Input: dimensioned drawing with shaded views. Units: mm. Origin: part minimum x, y, z. A direction names the side the tool comes from. Round coordinates to 2 decimals unless told otherwise and drop trailing zeros. Order: outer loops, then holes, each group sorted by start corner. A loop starts at its lowest first (then second) coordinate and runs counter-clockwise, first axis right, second up.
Item 1: Mould query, pull axis Z, two halves, no side actions, for the marked faces 3, 4 and 5. Classes: released by +Z, released by -Z, zero draft, split by the parting line, or undercut.
Item 2: Cut plane B-B on y = 38.1. Output: boundary loops of the cut face in (x, z), then the cut area to 3 significant figures.
Item 3: Cut plane D-D on z = 38.1. Output: boundary loops of the cut face in (x, y).
Item 4: Cut plane C-C on x = 22.86. Output: boundary loops of the cut face in (y, z), then the cut area to 3 significant figures.
Item 5: Cut plane A-A on z = 10.16. Output: boundary loops of the cut face in (x, y), then the cut area to 3 significant figures.
Item 6: Line query: L1, parallel to X at y = 6, z = 10; L2, parallel to Z at x = 78.74, y = 2.75; L3, parallel to X at y = 6.5, z = 67. Output: solid intervals per line, ascending.
Item 7: First-contact query: pin 1 (3 mm diameter, centred on x = 10.5, y = 66.5, fed in from +Z); pin 2 (2.5 mm diameter, centred on x = 22.86, z = 10.16, fed in from +Y); pin 3 (5 mm diameter, centred on x = 79, z = 63.5, fed in from +Y). Flat tips, straight axial feed; report the tip coordinate or a pass-through.
Item 8: Reachability of the marked faces 1 and 2 from +Z, -Z, +X, -X, +Y, -Y: full face, straight path, thin tool, end or side. Return the list, or none.
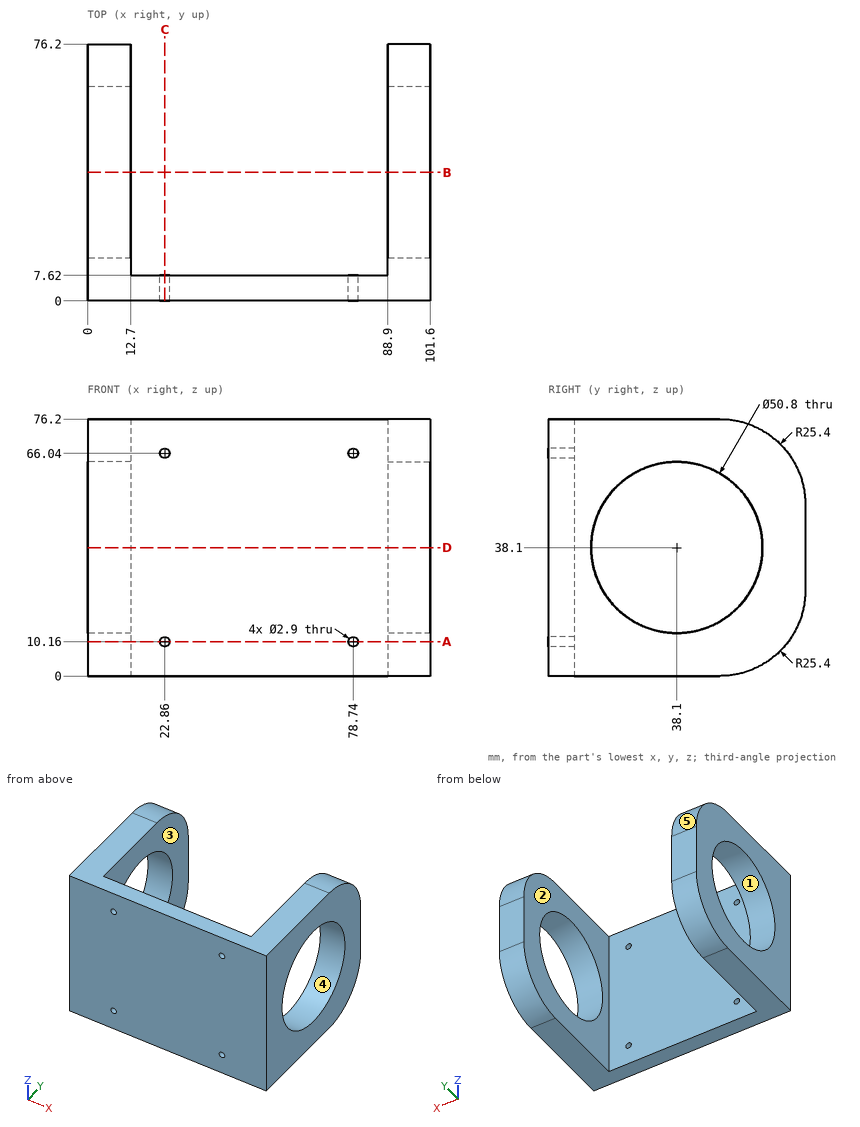
From the geometry:
1. face 3: zero draft
1. face 4: undercut
1. face 5: released by +Z
2. outline: (0, 0) - (12.7, 0) - (12.7, 12.7) - (0, 12.7) - close; (0, 63.5) - (12.7, 63.5) - (12.7, 76.2) - (0, 76.2) - close; (88.9, 0) - (101.6, 0) - (101.6, 12.7) - (88.9, 12.7) - close; (88.9, 63.5) - (101.6, 63.5) - (101.6, 76.2) - (88.9, 76.2) - close
2. area: 645 mm2
3. outline: (0, 0) - (101.6, 0) - (101.6, 12.7) - (88.9, 12.7) - (88.9, 7.62) - (12.7, 7.62) - (12.7, 12.7) - (0, 12.7) - close; (0, 63.5) - (12.7, 63.5) - (12.7, 76.2) - (0, 76.2) - close; (88.9, 63.5) - (101.6, 63.5) - (101.6, 76.2) - (88.9, 76.2) - close
4. outline: (0, 0) - (7.62, 0) - (7.62, 8.71) - (0, 8.71) - close; (0, 11.61) - (7.62, 11.61) - (7.62, 64.59) - (0, 64.59) - close; (0, 67.49) - (7.62, 67.49) - (7.62, 76.2) - (0, 76.2) - close
4. area: 536 mm2
5. outline: (0, 0) - (21.41, 0) - (21.41, 7.62) - (12.7, 7.62) - (12.7, 71.12) - (0, 71.12) - close; (24.31, 0) - (77.29, 0) - (77.29, 7.62) - (24.31, 7.62) - close; (80.19, 0) - (101.6, 0) - (101.6, 71.12) - (88.9, 71.12) - (88.9, 7.62) - (80.19, 7.62) - close
5. area: 2,340 mm2
6. L1: x = 0 to 21.42, 24.3 to 77.3, 80.18 to 101.6
6. L2: z = 0 to 8.71, 11.61 to 64.59, 67.49 to 76.2
6. L3: x = 0 to 21.77, 23.95 to 77.65, 79.83 to 101.6
7. pin 1: stops at z = 71.86
7. pin 2: passes through
7. pin 3: stops at y = 7.62
8. face 1: +X, -X
8. face 2: +Z, -Z, +Y
